Can you work these out from the drawing? Everything is in mm from the part's minimum corner. Coordinates: 2 decimals unless noted, no trailing zeros. Order: outer loops, then holes, each group sorted by start corner. A loop starts at its lowest first (then second) coordinate and runs counter-clockwise, first axis right, second up. Notation, with made-up numbers: (57.25, -33.5) -> (69.25, -33.5) arc R15 ccw to (69.25, -18.5) -> close; hole circle Ø6 at (49.5, -21). An arc over 180 degrees is marked (long way). Put each result on its own line as item: value. Start each with the question number.
Q1. Will this pin go through, and if not, where does the flat tip stop? pin 1 (4 mm diameter, centred on x = 7.4, z = 7.5, fed in from -Y).
Q2. If we section it at C-C (x = 62.5): Please give me the cut outline in (y, z), and give its area (3 significant figures).
Q3. If we section it at A-A (z = 41.5): Please give me the cut outline in (x, y), and give its area (3 significant figures).
Q4. If we section it at D-D (x = 42): Please give me the cut outline in (y, z).
Q5. Please list where these lines run through material, in increasing order: line 1 along X through (y, z) = (1.3, 7.5); line 2 along Z through (x, y) = (62.5, 0.8); line 3 along X through (y, z) = (1.95, 50).
Q6. If we section it at B-B (z = 60): Please give me the cut outline in (x, y).
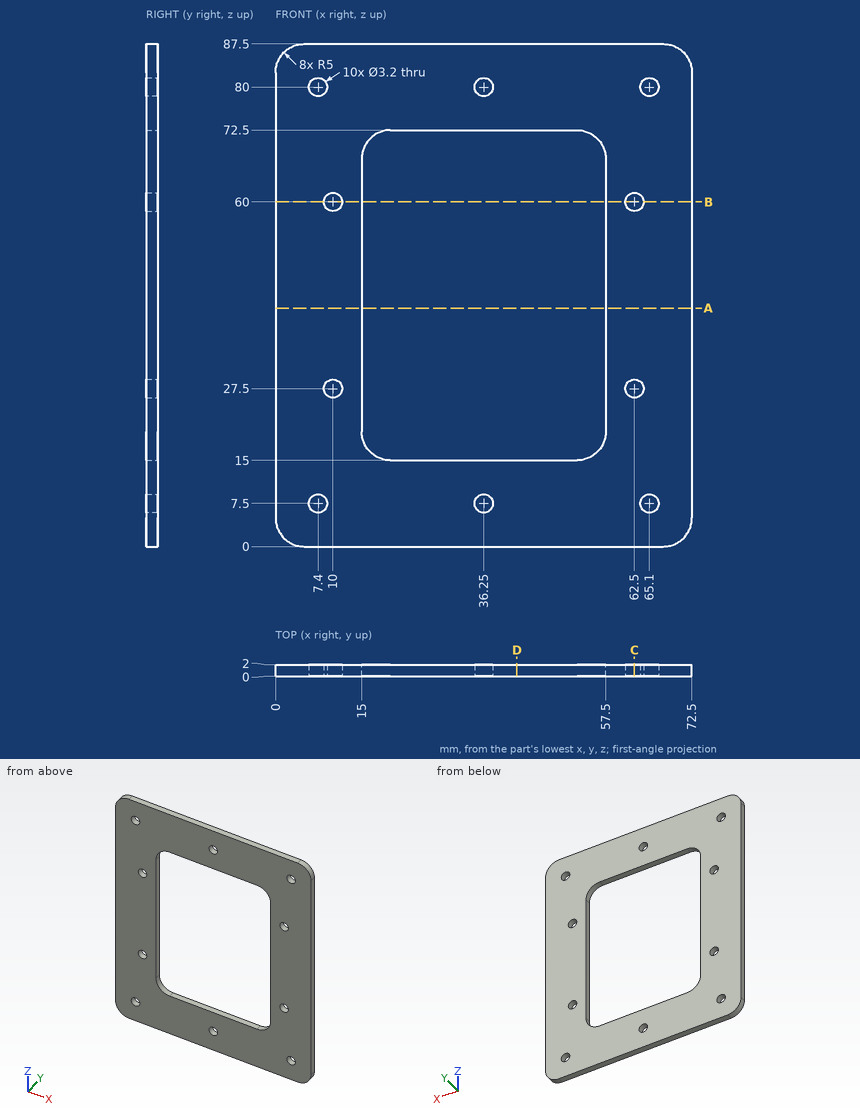
The answers:
1. pin 1: y = 0
2. outline: (0, 0) -> (2, 0) -> (2, 25.9) -> (0, 25.9) -> close; (0, 29.1) -> (2, 29.1) -> (2, 58.4) -> (0, 58.4) -> close; (0, 61.6) -> (2, 61.6) -> (2, 87.5) -> (0, 87.5) -> close
2. area: 162 mm^2
3. outline: (0, 0) -> (15, 0) -> (15, 2) -> (0, 2) -> close; (57.5, 0) -> (72.5, 0) -> (72.5, 2) -> (57.5, 2) -> close
3. area: 60.0 mm^2
4. outline: (0, 0) -> (2, 0) -> (2, 15) -> (0, 15) -> close; (0, 72.5) -> (2, 72.5) -> (2, 87.5) -> (0, 87.5) -> close
5. line 1: 0 to 5.8, 9 to 34.65, 37.85 to 63.5, 66.7 to 72.5
5. line 2: 0 to 25.9, 29.1 to 58.4, 61.6 to 87.5
5. line 3: 0 to 15, 57.5 to 72.5
6. outline: (0, 0) -> (8.4, 0) -> (8.4, 2) -> (0, 2) -> close; (11.6, 0) -> (15, 0) -> (15, 2) -> (11.6, 2) -> close; (57.5, 0) -> (60.9, 0) -> (60.9, 2) -> (57.5, 2) -> close; (64.1, 0) -> (72.5, 0) -> (72.5, 2) -> (64.1, 2) -> close
